For this review, take the finished solid that the model builds, in its own axes (mm). A direction names the side the tool comes from. Round coordinates to 2 decimals unless told otherwise and drop trailing zeros. Loops run counter-clockwise (first coordinate to the right, second up) from the corner with the lowest first, then second, coordinate; pieces in that order, holes last. Notation, with made-up numbers: (-23.5, -8.5) -> (18.5, -8.5) arc R19 ccw to (18.5, 1.5) -> close; hole circle Ø7 at (-6.75, 32). An arc over 180 degrees is marked (long way). One line per question, with ' | ' between items. Start each with the question number.
1. For pin 1 Ø4 at (x, z) = (70, 10) entering from -Y; pin 2 Ø7 at (x, z) = (10, 50) entering from -Y, all flat-tipped, find the tip position at first contact; note any pin that passes through.
2. For faces 1 (the face through (76, 2, 5)), 2 (the face through (22.86, 9.93, 44.59)), 3 (the face through (40, 7, 0)), list the 3-axis set-ups (+Z, -Z, +X, -X, +Y, -Y) from which the entire face can be reached by the end or side of a thin tool; tool diameter is ignored.
3. Consider section C-C (x = 62.5). Write out the cut boundary in (y, z), and give its area (3 significant figures).
4. Draft analysis for pull direction X (two halves, no side actions). For faces 4 (the face through (11.52, 9.93, 8.34)), 5 (the face through (40, 0, 1)), 6 (the face through (3.01, 7.4, 57.15)), state which applies: pulls with the +X half, pulls with the -X half, needs draft (parallel to the pull), parting line crosses it, or undercut.
5. Consider section A-A (z = 35). Write out the cut boundary in (x, y), and give its area (3 significant figures).
6. Wall thickness on line 1 along X through (y, z) = (9.25, 10); line 2 along Z through (x, y) = (70, 11.25); line 3 along Z through (x, y) = (36.5, 5.75): over which ranges is each line inside the solid? List them lowest first.
7. Consider section D-D (z = 4). Write out the cut boundary in (x, y).
8. Consider section B-B (y = 1.75). Write out the cut boundary in (x, z).
```python
from build123d import *

# Parameters (mm, degrees)
ESQUISSE1_R             = 2.25
BOSS_EXTRU_1_DEPTH      = 15
ENL_V_MAT_EXTRU_1_DEPTH = 5


with BuildPart() as part:
    # Esquisse1 → Boss.-Extru.1 (new body)
    with BuildSketch(Plane(origin=(0, 0, 0), x_dir=(1, 0, 0), z_dir=(0, 1, 0))):
        with BuildLine():
            Line((10, 0), (70, 0))
            ThreePointArc((70, 0), (77.071067812, -2.928932188), (80, -10))
            Line((80, -10), (80, -50))
            ThreePointArc((80, -50), (77.071067812, -57.071067812), (70, -60))
            Line((70, -60), (10, -60))
            ThreePointArc((10, -60), (2.928932188, -57.071067812), (0, -50))
            Line((0, -50), (0, -10))
            ThreePointArc((0, -10), (2.928932188, -2.928932188), (10, 0))
        make_face()
        with Locations(Location((10, -10, 0), (0, 0, 270))):
            Circle(ESQUISSE1_R, mode=Mode.SUBTRACT)
        with Locations(Location((70, -10, 0), (0, 0, 270))):
            Circle(ESQUISSE1_R, mode=Mode.SUBTRACT)
        with Locations(Location((10, -50, 0), (0, 0, 270))):
            Circle(ESQUISSE1_R, mode=Mode.SUBTRACT)
        with Locations(Location((70, -50, 0), (0, 0, 270))):
            Circle(ESQUISSE1_R, mode=Mode.SUBTRACT)
        with BuildLine():
            Line((24.253765099, -14.157246889), (57.253765099, -14.157246889))
            ThreePointArc((57.253765099, -14.157246889), (58.667978662, -14.743033326), (59.253765099, -16.157246889))
            Line((59.253765099, -16.157246889), (59.253765099, -43.157246889))
            ThreePointArc((59.253765099, -43.157246889), (58.667978662, -44.571460451), (57.253765099, -45.157246889))
            Line((57.253765099, -45.157246889), (24.253765099, -45.157246889))
            ThreePointArc((24.253765099, -45.157246889), (22.839551537, -44.571460451), (22.253765099, -43.157246889))
            Line((22.253765099, -43.157246889), (22.253765099, -16.157246889))
            ThreePointArc((22.253765099, -16.157246889), (22.839551537, -14.743033326), (24.253765099, -14.157246889))
        make_face(mode=Mode.SUBTRACT)
    extrude(amount=BOSS_EXTRU_1_DEPTH)

    # Esquisse2 → Enlèv. mat.-Extru.1 (cut)
    with BuildSketch(Plane.XZ):
        with BuildLine():
            Line((8, 57), (72, 57))
            ThreePointArc((72, 57), (75.535533906, 55.535533906), (77, 52))
            Line((77, 52), (77, 8))
            ThreePointArc((77, 8), (75.535533906, 4.464466094), (72, 3))
            Line((72, 3), (8, 3))
            ThreePointArc((8, 3), (4.464466094, 4.464466094), (3, 8))
            Line((3, 8), (3, 52))
            ThreePointArc((3, 52), (4.464466094, 55.535533906), (8, 57))
        make_face()
    extrude(amount=-ENL_V_MAT_EXTRU_1_DEPTH, mode=Mode.SUBTRACT)


solid = part.part
```
Answer block:
1) pin 1: passes through | pin 2: stops at y = 5
2) face 1: -Y | face 2: +Y, -Y | face 3: -Z, +X, -X, +Y, -Y
3) outline: (0, 0) -> (15, 0) -> (15, 60) -> (0, 60) -> (0, 57) -> (5, 57) -> (5, 3) -> (0, 3) -> close | area: 630 mm2
4) face 4: undercut | face 5: needs draft | face 6: pulls with the -X half
5) outline: (0, 0) -> (3, 0) -> (3, 5) -> (22.25, 5) -> (22.25, 15) -> (0, 15) -> close; (59.25, 5) -> (77, 5) -> (77, 0) -> (80, 0) -> (80, 15) -> (59.25, 15) -> close | area: 460 mm2
6) line 1: x = 0 to 7.75, 12.25 to 67.75, 72.25 to 80 | line 2: z = 0 to 7.75, 12.25 to 47.75, 52.25 to 60 | line 3: z = 0 to 14.16, 45.16 to 60
7) outline: (2, 0) -> (5, 0) -> (5, 5) -> (75, 5) -> (75, 0) -> (78, 0) -> (78, 15) -> (2, 15) -> close
8) outline: (0, 10) arc R10 ccw to (10, 0) -> (70, 0) arc R10 ccw to (80, 10) -> (80, 50) arc R10 ccw to (70, 60) -> (10, 60) arc R10 ccw to (0, 50) -> close; hole (3, 8) arc R5 ccw to (8, 3) -> (72, 3) arc R5 ccw to (77, 8) -> (77, 52) arc R5 ccw to (72, 57) -> (8, 57) arc R5 ccw to (3, 52) -> close
